Verification items for the finished model (mm, model axes). A direction names the side the tool comes from. Give positions to 0.01 mm unless a question says otherwise; leave off trailing zeros. Write each loop counter-clockwise with the first axis right and the second up, starting at its lowest first coordinate (ties: lowest second). Pieces come first, ordered by that corner, then holes. Notation, with made-up numbers: (58.25, 27.5) - (98.25, 27.5) arc R22 ccw to (98.25, 54.5) - close; hole circle Ø5 at (-33.5, 34.5). An arc over 180 degrees is marked (long way). Answer as a JSON object with one key per item and string values. Group by question number.
Item 1: Draft check along X on faces 3 (the face through (-1.032, 4.647, -11.371)), 4 (the face through (0, 0, -18.415)), 5 (the face through (-2.4, -1.4, -0.2)). Enter one of: +X half, -X half, draft (parallel to the pull), parting line (faces both ways), or undercut.
Item 2: Sectioned sample at A-A, the plane z = -7.25. Record the boundary of the cut face in (x, y), and give its area (3 significant figures).
Item 3: Tool access check on faces 1 (the face through (-2.4, 1.4, -0.2)), 2 (the face through (-4.86, -1.08, -2.54)). Record the directions out of +Z, -Z, +X, -X, +Y, -Y that give a thin tool (end or side, any length) a straight path to the whole face; none if there is none.
Item 4: Go/stop test with flat-tipped pins: pin 1 (2 mm diameter, centred on y = 0.5, z = -3.5, fed in from +X); pin 2 (3 mm diameter, centred on x = 1.5, y = 1.5, fed in from +Z); pin 3 (3.5 mm diameter, centred on x = 0, z = -0.5, fed in from +Y); pin 4 (1 mm diameter, centred on x = -6, z = -1, fed in from -Y). Record where each tip stops, or that it passes through.
Item 5: Scan lines: line 1 along X through (y, z) = (-0.25, -13); line 2 along Y through (x, z) = (3, 0.25). Record each from-to range of solid material in increasing order. Write a range as [from, to].
Solid Edge part; units mm, degrees
sketch "Sketch1" plane through (0, 0, 0) normal (1, 0, 0) x (0, 1, 0)
  line L0 (0, -2.54) -> (0, 2.54)
  arc A0 (0, 2.54) -> (8.255, -2.54) centre (-0.5525, -7.605) cw
  line L1 (0, -2.54) -> (8.255, -2.54)
revolve "RevolvedProtrusion1" add sketch "Sketch1" angle 360 about axis through (0, 0, -14.7796) along (0, 0, 1)
sketch "Sketch2" plane through (0, 0, -2.54) normal (0, 0, -1) x (0, 1, 0)
  circle A0 centre (0, 0) radius 4.7625
extrude "Protrusion1" add sketch "Sketch2" along normal blind 15.875
sketch "Sketch3" plane through (0, 0, -18.415) normal (0, 0, -1) x (1, 0, 0)
  circle A0 centre (0, 0) radius 4.76
extrude "Cutout1" cut sketch "Sketch3" against normal blind 14.2875 flip side to cut
sketch "Sketch4" plane through (-0.6032, 0.3606, 5.08) normal (0, 0, 1) x (1, 0, 0)
  line L0 (-1.0007, 2.4175) -> (2.2072, 2.4175)
  line L1 (3.8111, -0.3606) -> (2.2072, 2.4175)
  line L2 (2.2072, -3.1387) -> (3.8111, -0.3606)
  line L3 (-1.0007, -3.1387) -> (2.2072, -3.1387)
  line L4 (-2.6047, -0.3606) -> (-1.0007, -3.1387)
  line L5 (-1.0007, 2.4175) -> (-2.6047, -0.3606)
extrude "ExtrudedCutout_11" cut sketch "Sketch4" against normal blind 7.62
properties part number "163739"
Geometry check:
{
 "1": {"face 3": "parting line", "face 4": "draft", "face 5": "undercut"},
 "2": {"outline": "circle Ø9.52 at (0, 0)", "area": "71.2 mm^2"},
 "3": {"face 1": "+Z", "face 2": "-Z"},
 "4": {"pin 1": "x = 8.25", "pin 2": "z = 1.99", "pin 3": "y = 8.08", "pin 4": "y = -4.87"},
 "5": {"line 1": "[-4.75, 4.75]", "line 2": "[-5.07, -0.36], [0.36, 5.07]"}
}
